Read the model definition and answer for the solid it produces. Units are mm, in the model's axes. A direction names the side the tool comes from. Round coordinates to 2 decimals unless told otherwise and drop trailing zeros. Order: outer loops, then holes, each group sorted by start corner. A loop starts at its lowest first (then second) coordinate and runs counter-clockwise, first axis right, second up. Notation, with made-up numbers: (2.25, 48) -> (19.25, 48) arc R11 cw to (19.25, 62) -> close; hole circle Ø4 at (-14, 26.5). An arc over 180 degrees is marked (long way). Use a Markdown table: item, result. Add a question column.
1. Section B-B, the plane y = 84.5 is taken. Give the vertices of the cut face in (x, z).
2. Given pin 1 (1 mm diameter, centred on x = -16, y = 55.5, fed in from +Z); pin 2 (2.5 mm diameter, centred on y = 228.5, z = -1, fed in from -X); pin 3 (4.5 mm diameter, centred on y = 241.59, z = 0, fed in from +X), each flat-ended and moving along its own axis, determine where each tip first touches the part or whether it passes through.
3. The mould has two halves that part along Y. Classify faces 5 (the face through (0, 254, -11)), 6 (the face through (0, 12, -23.812)), 7 (the face through (23.812, 125, 13)): +Y half, -Y half, draft (parallel to the pull), parting line (faces both ways), or undercut.
4. Consider L1, parallel to X at y = 236, z = 5; L2, parallel to X at y = 228.6, z = -24.9 (3 decimals); L3, parallel to Y at x = 0, z = -24.9 (3 decimals). Determine where each line is inside the solid, lowest interval first. Write a range as [from, to].
5. For faces 1 (the face through (23.812, 242, 0)), 2 (the face through (0, 242, -23.812)), 3 (the face through (-23.812, 125, 13)), 4 (the face through (-24.595, 239.245, 0.52)), determine the directions among +Z, -Z, +X, -X, +Y, -Y from which every point of the face is accessible in a straight line to the end or side of a thin tool.
6. Section C-C, the plane x = 0 is taken. Give the vertices of the cut face in (y, z) (1 decimal), then the cut area to 3 significant figures.
7. Section A-A, the plane z = 10.5 is taken. Give the vertices of the cut face in (x, y).
8. Section D-D, the plane y = 228.6 is taken. Give the vertices of the cut face in (x, z) (1 decimal).
```python
from build123d import *

# Parameters (mm, degrees)
SKETCH1_W               = 50.8
SKETCH1_H               = 50.8
SKETCH1_W_2             = 47.625
SKETCH1_H_2             = 47.625
BOSS_EXTRUDE1_DEPTH     = 254
SKETCH4_R               = 2.3999952
CUT_EXTRUDE1_DEPTH      = 50.2125
CUT_EXTRUDE1_DEPTH_BACK = 2.5875
SKETCH5_R               = 2.3999952
CUT_EXTRUDE2_DEPTH      = 51.8
SKETCH6_R               = 2.3999952
CUT_EXTRUDE3_DEPTH      = 1
CUT_EXTRUDE3_DEPTH_BACK = 51.8
SKETCH7_R               = 2.3999952
CUT_EXTRUDE4_DEPTH      = 1
CUT_EXTRUDE4_DEPTH_BACK = 51.8
SKETCH8_R               = 3.175
CUT_EXTRUDE5_DEPTH      = 1
CUT_EXTRUDE5_DEPTH_BACK = 51.8
SKETCH9_R               = 3.175
CUT_EXTRUDE6_DEPTH      = 1
CUT_EXTRUDE6_DEPTH_BACK = 51.8
CUT_EXTRUDE7_REACH      = 256
SKETCH10_W              = 47.625
SKETCH10_H              = 1.5875
SKETCH11_W              = 47.625
SKETCH11_H              = 25.4
BOSS_EXTRUDE2_DEPTH     = 254


with BuildPart() as part:
    # Sketch1 → Boss-Extrude1 (new body)
    with BuildSketch(Plane(origin=(0, 0, 0), x_dir=(1, 0, 0), z_dir=(0, 1, 0))):
        Rectangle(SKETCH1_W, SKETCH1_H)
        Rectangle(SKETCH1_W_2, SKETCH1_H_2, mode=Mode.SUBTRACT)
    extrude(amount=BOSS_EXTRUDE1_DEPTH)

    # Sketch4 → Cut-Extrude1 (cut, two sides)
    with BuildSketch(Plane(origin=(-23.8125, 0, 0), x_dir=(0, 0, -1), z_dir=(1, 0, 0))) as cut_extrude1_sk:
        with Locations((0, 241.587599882)):
            Circle(SKETCH4_R)
    extrude(amount=CUT_EXTRUDE1_DEPTH, mode=Mode.SUBTRACT)
    extrude(cut_extrude1_sk.sketch, amount=-CUT_EXTRUDE1_DEPTH_BACK, mode=Mode.SUBTRACT)

    # Sketch5 → Cut-Extrude2 (cut, through all)
    with BuildSketch(Plane(origin=(0, 0, -25.4), x_dir=(-1, 0, 0), z_dir=(0, 0, -1))):
        with Locations((0, 241.587599882)):
            Circle(SKETCH5_R)
    extrude(amount=-CUT_EXTRUDE2_DEPTH, mode=Mode.SUBTRACT)

    # Sketch6 → Cut-Extrude3 (cut, two sides)
    with BuildSketch(Plane(origin=(25.4, 0, 0), x_dir=(0, 0, -1), z_dir=(1, 0, 0))) as cut_extrude3_sk:
        with Locations((0, 12.412400118)):
            Circle(SKETCH6_R)
    extrude(amount=CUT_EXTRUDE3_DEPTH, mode=Mode.SUBTRACT)
    extrude(cut_extrude3_sk.sketch, amount=-CUT_EXTRUDE3_DEPTH_BACK, mode=Mode.SUBTRACT)

    # Sketch7 → Cut-Extrude4 (cut, two sides)
    with BuildSketch(Plane(origin=(0, 0, -25.4), x_dir=(-1, 0, 0), z_dir=(0, 0, -1))) as cut_extrude4_sk:
        with Locations((0, 12.412400118)):
            Circle(SKETCH7_R)
    extrude(amount=CUT_EXTRUDE4_DEPTH, mode=Mode.SUBTRACT)
    extrude(cut_extrude4_sk.sketch, amount=-CUT_EXTRUDE4_DEPTH_BACK, mode=Mode.SUBTRACT)

    # Sketch8 → Cut-Extrude5 (cut, two sides)
    with BuildSketch(Plane(origin=(0, 0, -25.4), x_dir=(-1, 0, 0), z_dir=(0, 0, -1))) as cut_extrude5_sk:
        with Locations((0, 228.6)):
            Circle(SKETCH8_R)
    extrude(amount=CUT_EXTRUDE5_DEPTH, mode=Mode.SUBTRACT)
    extrude(cut_extrude5_sk.sketch, amount=-CUT_EXTRUDE5_DEPTH_BACK, mode=Mode.SUBTRACT)

    # Sketch9 → Cut-Extrude6 (cut, two sides)
    with BuildSketch(Plane(origin=(25.4, 0, 0), x_dir=(0, 0, -1), z_dir=(1, 0, 0))) as cut_extrude6_sk:
        with Locations((0, 228.6)):
            Circle(SKETCH9_R)
    extrude(amount=CUT_EXTRUDE6_DEPTH, mode=Mode.SUBTRACT)
    extrude(cut_extrude6_sk.sketch, amount=-CUT_EXTRUDE6_DEPTH_BACK, mode=Mode.SUBTRACT)

    # Sketch10 → Cut-Extrude7 (cut, up to next)
    with BuildSketch(Plane.XZ, mode=Mode.PRIVATE) as cut_extrude7_sk1:
        with Locations((0, 24.60625)):
            Rectangle(SKETCH10_W, SKETCH10_H)
    cut_extrude7_tool1 = extrude(cut_extrude7_sk1.sketch, amount=-CUT_EXTRUDE7_REACH, mode=Mode.PRIVATE) & part.part
    add(cut_extrude7_tool1.solids().sort_by_distance((0, 0, 24.60625))[0], mode=Mode.SUBTRACT)

    # Sketch11 → Boss-Extrude2 (add, through all)
    with BuildSketch(Plane.XZ):
        with Locations((0, -11.1125)):
            Rectangle(SKETCH11_W, SKETCH11_H)
    extrude(amount=-BOSS_EXTRUDE2_DEPTH)


solid = part.part
```
Verdict:
| question | item | result |
|---|---|---|
| 1 | outline | (-25.4, -25.4) -> (25.4, -25.4) -> (25.4, 25.4) -> (23.81, 25.4) -> (23.81, 1.59) -> (-23.81, 1.59) -> (-23.81, 25.4) -> (-25.4, 25.4) -> close |
| 2 | pin 1 | stops at z = 1.59 |
| 2 | pin 2 | stops at x = -23.81 |
| 2 | pin 3 | stops at x = 23.81 |
| 3 | face 5 | +Y half |
| 3 | face 6 | undercut |
| 3 | face 7 | draft |
| 4 | L1 | x = [-25.4, -23.81], [23.81, 25.4] |
| 4 | L2 | x = [-25.4, -3.175], [3.175, 25.4] |
| 4 | L3 | y = [0, 10.012], [14.812, 225.425], [231.775, 239.188], [243.988, 254] |
| 5 | face 1 | +X |
| 5 | face 2 | -Z |
| 5 | face 3 | +Z, +Y, -Y |
| 5 | face 4 | -X |
| 6 | outline | (0, -25.4) -> (10, -25.4) -> (10, -23.8) -> (14.8, -23.8) -> (14.8, -25.4) -> (225.4, -25.4) -> (225.4, -23.8) -> (231.8, -23.8) -> (231.8, -25.4) -> (239.2, -25.4) -> (239.2, -23.8) -> (244, -23.8) -> (244, -25.4) -> (254, -25.4) -> (254, 1.6) -> (0, 1.6) -> close |
| 6 | area | 6,830 mm2 |
| 7 | outline | (-25.4, 0) -> (-23.81, 0) -> (-23.81, 254) -> (-25.4, 254) -> close; (23.81, 0) -> (25.4, 0) -> (25.4, 254) -> (23.81, 254) -> close |
| 8 | outline | (-25.4, -25.4) -> (-3.2, -25.4) -> (-3.2, -23.8) -> (3.2, -23.8) -> (3.2, -25.4) -> (25.4, -25.4) -> (25.4, -3.2) -> (23.8, -3.2) -> (23.8, 1.6) -> (-23.8, 1.6) -> (-23.8, -3.2) -> (-25.4, -3.2) -> close; (-25.4, 3.2) -> (-23.8, 3.2) -> (-23.8, 25.4) -> (-25.4, 25.4) -> close; (23.8, 3.2) -> (25.4, 3.2) -> (25.4, 25.4) -> (23.8, 25.4) -> close |
